Build history of the part. All positions in model axes, mm. A direction names the side the tool comes from. Round coordinates to 2 decimals unless told otherwise and drop trailing zeros. Write each loop counter-clockwise with the first axis right and the second up, starting at its lowest first coordinate (ties: lowest second). Pieces come first, ordered by that corner, then holes. Notation, with made-up numbers: (76, -20) - (130, -20) arc R11 cw to (130, -5) - close; hole circle Ø7 at (89, 32.5). An arc over 180 degrees is marked (long way). One line per question, with ' | ' between items.
Autodesk Inventor part; units mm, degrees
ref_plane "Work Plane1" through (-12.8329, -37.377, 0) normal (-1, 0, 0) x (0, 0, 1)
ref_plane "Work Plane4" through (-12.8329, -29.5246, 6.35) normal (0, 0, 1) x (1, 0, 0)
ref_plane "YZ Plane" through (0, 0, 0) normal (1, 0, 0) x (0, 1, 0)
sketch "Sketch1" plane through (0, 0, 0) normal (0, 0, 1) x (1, 0, 0)
  circle A0 centre (-12.8329, -29.5246) radius 6.35
  line L0 (-6.0325, -33.4508) -> (-12.8329, -37.377)
  line L1 (-12.8329, -37.377) -> (-19.6333, -33.4508)
  line L2 (-19.6333, -33.4508) -> (-19.6333, -25.5984)
  line L3 (-19.6333, -25.5984) -> (-12.8329, -21.6722)
  line L4 (-12.8329, -21.6722) -> (-6.0325, -25.5984)
  line L5 (-6.0325, -25.5984) -> (-6.0325, -33.4508)
  circle A1 centre (-12.8329, -29.5246) radius 4.3656
  circle A2 centre (-12.8329, -29.5246) radius 6.35
  circle A3 centre (-12.8329, -29.5246) radius 6.8004
  line L6 (-12.8329, -21.6722) -> (-12.8329, -22.7242) construction
  dimension "d36" = 13.6008
  dimension "d37" = 1.052
extrude "Extrusion1" add sketch "Sketch1" along normal blind 12.7 contours A0 | L0 A3 L5 | L0 L1 A3 | A3 | A3 L4 L5 | L1 L2 A3 | A3 L3 L4 | L2 L3 A3 | A1
ref_plane "Work Plane1" through (-12.8329, -37.377, 0) normal (-1, 0, 0) x (0, 0, 1)
extrude "Extrusion3" add sketch "Sketch1" against normal blind 6.35 draft -1.783 contours A1
thread "Thread2"
sketch "Sketch6" plane through (0, 0, 12.7) normal (0, 0, 1) x (1, 0, 0)
  circle A0 centre (-12.8329, -29.5246) radius 6.35
  point P0 (0, 0)
hole "Hole2" at (-12.8329, -29.5246, 12.7) direction (0, 0, -1) diameter 3.302 end through all
sketch "Sketch7" plane through (0, 0, 12.7) normal (0, 0, 1) x (1, 0, 0)
  circle A0 centre (-12.8329, -29.5246) radius 1.651
  circle A1 centre (-12.8329, -29.5246) radius 4.3656
  point P0 (0, 0)
extrude "Extrusion4" add sketch "Sketch7" along normal blind 6.35 draft -1.783
thread "Thread3"
sketch "Sketch8" plane through (-12.8329, -37.377, 0) normal (-1, 0, 0) x (0, 0, 1)
  line L0 (12.7, 14.6507) -> (12.3564, 15.7048)
  line L1 (12.3564, 15.7048) -> (12.7, 14.6507)
  line L2 (12.3564, 15.7048) -> (12.7, 15.7048)
  line L3 (12.7, 15.7048) -> (12.7, 14.6507)
  line L4 (12.7, 15.7048) -> (12.7, 11.7786)
  line L5 (16.6116, 7.8524) -> (-10.7696, 7.8524)
  point P0 (0, 37.377)
  point P1 (-6.858, -1.905)
  dimension "d38" = 1.0541
revolve "Revolution3" cut sketch "Sketch8" angle 360 about axis through (-12.8329, -29.5246, 0) along (0, 0, -1)
ref_plane "Work Plane4" through (-12.8329, -29.5246, 6.35) normal (0, 0, 1) x (1, 0, 0)
mirror "Mirror4" about plane through (-12.8329, -29.5246, 6.35) normal (0, 0, 1) of "Revolution3"
properties part number "Pneumatic_VIAIR_Fitting"
Q1. Saw through at A-A, the plane z = 10.75. List the corners of the cut face in (x, y), then the cut area to 3 significant figures.
Found:
outline: (-19.63, -33.45) - (-12.83, -37.38) - (-6.03, -33.45) - (-6.03, -25.6) - (-12.83, -21.67) - (-19.63, -25.6) - close; hole circle Ø3.3 at (-12.83, -29.52) | area: 152 mm^2
Q2. Pull direction Y, two halves, no side cores. Call faces 4 (the conical face through (-13.213, -31.234, 15.919)), 5 (the cylindrical face through (-12.905, -27.875, 3.042)), 6 (the flat face through (-19.633, -30, 6)), 7 (the conical face through (-8.89, -31.16, -3.13)): +Y half, -Y half, draft (parallel to the pull), parting line (faces both ways), or undercut.
Found:
face 4: undercut | face 5: undercut | face 6: draft | face 7: parting line
Q3. Drop a flat-ended pin along its axis: pin 1 (4 mm diameter, centred on y = -29.5, z = -3, fed in from +X). Give the stop position or say it passes through.
Found:
pin 1: x = -8.5
Q4. Drill centre lines: L1, parallel to Z at x = -9.25, y = -26; L2, parallel to Y at x = -12, z = 2.5; L3, parallel to X at y = -31, z = 1. Where is each one in solid material? Low to high. Write a range as from..to.
Found:
L1: 0..12.7 | L2: -36.9..-30.95, -28.1..-22.15 | L3: -19.63..-13.57, -12.09..-6.03
Q5. Saw through at B-B, the plane z = -2. List the corners of the cut face in (x, y), then the cut area to 3 significant figures.
Found:
outline: circle Ø8.61 at (-12.83, -29.52); hole circle Ø3.3 at (-12.83, -29.52) | area: 49.6 mm^2
Q6. Which spindle directions (+Z, -Z, +X, -X, +Y, -Y) get a long thin tool onto all of the face, cutting with end or side? Do faces 1 (the flat face through (-8, -29, 0)), 2 (the conical face through (-10.5, -33.1, 15.8)), 3 (the flat face through (-16.19, -35.44, 6.26)). Say none if no direction does.
Found:
face 1: -Z | face 2: +Z | face 3: +Z, -Z, -X, -Y
